Check sheet for the modelled part. Datum: model origin and axes. Units: mm. A direction names the side the tool comes from. Round coordinates to 2 decimals unless told otherwise and drop trailing zeros. Write each loop counter-clockwise with the first axis right and the second up, starting at its lowest first coordinate (ties: lowest second). Pieces come first, ordered by that corner, then holes.
Item 1: Material ranges on line 1 along Z through (x, y) = (-65, 16.75); line 2 along X through (y, z) = (6.5, -20.5); line 3 along X through (y, z) = (1, -19), recorded low to high.
Item 2: Set-up check for faces 4 (the flat face through (17, 7, -5)), 5 (the cylindrical face through (-70.198, 14.698, 16.524)), 6 (the flat face through (75, 15, -25)), 7 (the flat face through (-52, 15, 21.5)), 8 (the flat face through (-66, 16, 6)): record each of +Z, -Z, +X, -X, +Y, -Y from which the full face is reachable in a straight line by a thin tool's end or side.
Item 3: Section check C-C, the plane x = -20. Record the cut outline in (y, z), plus the area to 3 significant figures.
Item 4: Section check B-B, the plane y = 5.25. Record the cut outline in (x, z).
Item 5: Release check for a two-part mould opening along Z. For faces 1 (the flat face through (-66.5, 14, -13)), 2 (the cylindrical face through (99.948, 7.395, 16.128)), 3 (the flat face through (-18, 9, 26.5)) record: pulls with the +Z half, pulls with the -Z half, needs draft (parallel to the pull), parting line crosses it, or undercut.
Item 6: Section check A-A, the plane x = 1. Record the cut outline in (y, z).
Item 7: Depth check by flat-ended pin: pin 1 (9.5 mm diameter, centred on y = 17.5, z = 14.5, fed in from +X); pin 2 (5 mm diameter, centred on y = 13, z = 5.5, fed in from +X); pin 3 (10 mm diameter, centred on x = -6, y = 12.5, fed in from -Z). Enter the tip coordinate at first touch or a pass-through.
from build123d import *

# Parameters (mm, degrees)
BOSS_EXTRUDE1_DEPTH      = 10
SKETCH3_W                = 10
SKETCH3_H                = 17
BOSS_EXTRUDE2_DEPTH      = 12.5
RIB1_REACH               = 118.391
SKETCH4_WALL_W           = 271.329674284
SKETCH4_WALL_H           = 5
CUT_EXTRUDE1_REACH       = 170.771
SKETCH6_R                = 2.55
CUT_EXTRUDE2_DEPTH       = 2.5
BOSS_EXTRUDE4_DEPTH      = 5
BOSS_EXTRUDE4_DEPTH_BACK = 10
SKETCH11_R               = 30
CUT_EXTRUDE3_REACH       = 111.582
SKETCH8_R                = 14
CUT_EXTRUDE4_DEPTH       = 6
CUT_EXTRUDE4_DEPTH_BACK  = 7
SKETCH9_R                = 18.5
SKETCH12_R               = 24.5
CUT_EXTRUDE6_DEPTH       = 6
SKETCH13_R               = 2.05
CUT_EXTRUDE7_DEPTH       = 110.581884276
CUT_EXTRUDE9_START       = -2
SKETCH15_R               = 24.5
CUT_EXTRUDE9_DEPTH       = 2
SKETCH17_R               = 11.1
CUT_EXTRUDE11_DEPTH      = 7
CUT_EXTRUDE12_REACH      = 111.964
SKETCH18_R               = 4.5
SKETCH19_R               = 11.1
CUT_EXTRUDE13_DEPTH      = 7
CUT_EXTRUDE14_REACH      = 111.964
SKETCH20_R               = 4.5
SKETCH21_W               = 7
SKETCH21_H               = 3
BOSS_EXTRUDE5_DEPTH      = 7
SKETCH22_W               = 7
SKETCH22_H               = 2
BOSS_EXTRUDE6_DEPTH      = 5
SKETCH23_W               = 9.67527482
SKETCH23_H               = 3
BOSS_EXTRUDE7_DEPTH      = 8
SKETCH24_W               = 9.67527482
SKETCH24_H               = 2
BOSS_EXTRUDE8_DEPTH      = 3


with BuildPart() as part:
    # Sketch2 → Boss-Extrude1 (new body)
    with BuildSketch(Plane(origin=(0, 0, 0), x_dir=(1, 0, 0), z_dir=(0, 1, 0))):
        with BuildLine():
            Line((-74, 26.5), (74.6515139, 26.5))
            ThreePointArc((74.6515139, 26.5), (101.1515139, 0), (74.6515139, -26.5))
            Line((74.6515139, -26.5), (-74, -26.5))
            Line((-74, -26.5), (-74, 26.5))
        make_face()
    extrude(amount=BOSS_EXTRUDE1_DEPTH)

    # Sketch3 → Boss-Extrude2 (add)
    with BuildSketch(Plane(origin=(0, 10, 0), x_dir=(1, 0, 0), z_dir=(0, 1, 0))):
        with Locations((-69, -18)):
            Rectangle(SKETCH3_W, SKETCH3_H)
        with Locations((-69, 18)):
            Rectangle(SKETCH3_W, SKETCH3_H)
    extrude(amount=BOSS_EXTRUDE2_DEPTH)

    # Sketch4 wall → Rib1 (add, up to next)
    with BuildSketch(Plane(origin=(-46.828266128, 16.25, 26.5), x_dir=(0.939692620785, -0.342020143327, 0), z_dir=(0.342020143327, 0.939692620785, 0)), mode=Mode.PRIVATE) as rib1_sk1:
        with Locations((0, 2.5)):
            Rectangle(SKETCH4_WALL_W, SKETCH4_WALL_H)
    rib1_tool1 = extrude(rib1_sk1.sketch, amount=-RIB1_REACH, mode=Mode.PRIVATE) - part.part
    rib1 = rib1_tool1.solids().sort_by_distance((-46.828266128, 16.25, 26.5))[0]
    add(rib1)

    # Mirror1: Rib1 across plane
    add(rib1.mirror(Plane.XY))

    # Sketch6 → Cut-Extrude1 (cut, up to next)
    with BuildSketch(Plane(origin=(-64, 0, 0), x_dir=(0, 0, -1), z_dir=(1, 0, 0)), mode=Mode.PRIVATE) as cut_extrude1_sk1:
        with Locations((-14.5, 16.25)):
            Circle(SKETCH6_R)
    cut_extrude1_tool1 = extrude(cut_extrude1_sk1.sketch, amount=-CUT_EXTRUDE1_REACH, mode=Mode.PRIVATE) & part.part
    cut_extrude1 = cut_extrude1_tool1.solids().sort_by_distance((-64, 16.25, 14.5))[0]
    add(cut_extrude1, mode=Mode.SUBTRACT)

    # Sketch7 → Cut-Extrude2 (cut)
    with BuildSketch(Plane(origin=(-64, 0, 0), x_dir=(0, 0, -1), z_dir=(1, 0, 0))):
        Polygon((-10.45, 13.91173141), (-10.45, 18.58826859), (-14.5, 20.92653718), (-18.55, 18.58826859), (-18.55, 13.91173141), (-14.5, 11.57346282), align=None)
    cut_extrude2 = extrude(amount=-CUT_EXTRUDE2_DEPTH, mode=Mode.SUBTRACT)

    # Mirror2: Cut-Extrude1, Cut-Extrude2 across plane
    add(cut_extrude1.mirror(Plane.XY), mode=Mode.SUBTRACT)
    add(cut_extrude2.mirror(Plane.XY), mode=Mode.SUBTRACT)

    # Sketch11 → Boss-Extrude4 (add, two sides: drawn at the far end of the back side and taken through both)
    with BuildSketch(Plane(origin=(0, 10, 0), x_dir=(1, 0, 0), z_dir=(0, 1, 0)).offset(-BOSS_EXTRUDE4_DEPTH_BACK)):
        with Locations(Location((74.6515139, 0, 0), (0, 0, 270))):
            Circle(SKETCH11_R)
    extrude(amount=BOSS_EXTRUDE4_DEPTH + BOSS_EXTRUDE4_DEPTH_BACK)

    # Sketch8 → Cut-Extrude3 (cut, up to next)
    with BuildSketch(Plane(origin=(0, 10, 0), x_dir=(1, 0, 0), z_dir=(0, 1, 0)), mode=Mode.PRIVATE) as cut_extrude3_sk1:
        with Locations(Location((74.6515139, 0, 0), (0, 0, 270))):
            Circle(SKETCH8_R)
    cut_extrude3_tool1 = extrude(cut_extrude3_sk1.sketch, amount=-CUT_EXTRUDE3_REACH, mode=Mode.PRIVATE) & part.part
    add(cut_extrude3_tool1.solids().sort_by_distance((74.651514, 10, 0))[0], mode=Mode.SUBTRACT)

    # Sketch9 → Cut-Extrude4 (cut, two sides: drawn at the far end of the back side and taken through both)
    with BuildSketch(Plane(origin=(0, 10, 0), x_dir=(1, 0, 0), z_dir=(0, 1, 0)).offset(-CUT_EXTRUDE4_DEPTH_BACK)):
        with Locations(Location((74.6515139, 0, 0), (0, 0, 270))):
            Circle(SKETCH9_R)
    extrude(amount=CUT_EXTRUDE4_DEPTH + CUT_EXTRUDE4_DEPTH_BACK, mode=Mode.SUBTRACT)

    # Sketch12 → Cut-Extrude6 (cut)
    with BuildSketch(Plane(origin=(0, 15, 0), x_dir=(1, 0, 0), z_dir=(0, 1, 0))):
        with Locations(Location((74.6515139, 0, 0), (0, 0, 270))):
            Circle(SKETCH12_R)
    extrude(amount=-CUT_EXTRUDE6_DEPTH, mode=Mode.SUBTRACT)

    # Sketch13 → Cut-Extrude7 (cut, through all)
    with BuildSketch(Plane(origin=(0, 10, 0), x_dir=(1, 0, 0), z_dir=(0, 1, 0))):
        with Locations(Location((1, -20.5, 0), (0, 0, 270))):
            Circle(SKETCH13_R)
        with Locations(Location((31, -20.5, 0), (0, 0, 270))):
            Circle(SKETCH13_R)
    cut_extrude7 = extrude(amount=-CUT_EXTRUDE7_DEPTH, mode=Mode.SUBTRACT)

    # Sketch15 → Cut-Extrude9 (cut)
    with BuildSketch(Plane.XZ.offset(CUT_EXTRUDE9_START)):
        with Locations(Location((74.6515139, 0, 0), (0, 0, 90))):
            Circle(SKETCH15_R)
    extrude(amount=CUT_EXTRUDE9_DEPTH, mode=Mode.SUBTRACT)

    # Sketch17 → Cut-Extrude11 (cut)
    with BuildSketch(Plane.XZ):
        with Locations(Location((-40.5, 0, 0), (0, 0, 270))):
            Circle(SKETCH17_R)
    extrude(amount=-CUT_EXTRUDE11_DEPTH, mode=Mode.SUBTRACT)

    # Sketch18 → Cut-Extrude12 (cut, up to next)
    with BuildSketch(Plane.XZ.offset(-7), mode=Mode.PRIVATE) as cut_extrude12_sk1:
        with Locations(Location((-40.5, 0, 0), (0, 0, 270))):
            Circle(SKETCH18_R)
    cut_extrude12_tool1 = extrude(cut_extrude12_sk1.sketch, amount=-CUT_EXTRUDE12_REACH, mode=Mode.PRIVATE) & part.part
    add(cut_extrude12_tool1.solids().sort_by_distance((-40.5, 7, 0))[0], mode=Mode.SUBTRACT)

    # Sketch19 → Cut-Extrude13 (cut)
    with BuildSketch(Plane.XZ):
        with Locations(Location((17, 0, 0), (0, 0, 270))):
            Circle(SKETCH19_R)
    extrude(amount=-CUT_EXTRUDE13_DEPTH, mode=Mode.SUBTRACT)

    # Sketch20 → Cut-Extrude14 (cut, up to next)
    with BuildSketch(Plane.XZ.offset(-7), mode=Mode.PRIVATE) as cut_extrude14_sk1:
        with Locations(Location((17, 0, 0), (0, 0, 270))):
            Circle(SKETCH20_R)
    cut_extrude14_tool1 = extrude(cut_extrude14_sk1.sketch, amount=-CUT_EXTRUDE14_REACH, mode=Mode.PRIVATE) & part.part
    add(cut_extrude14_tool1.solids().sort_by_distance((17, 7, 0))[0], mode=Mode.SUBTRACT)

    # Mirror3: Cut-Extrude7 across plane
    add(cut_extrude7.mirror(Plane.XY), mode=Mode.SUBTRACT)

    # Sketch21 → Boss-Extrude5 (add)
    with BuildSketch(Plane(origin=(0, 10, 0), x_dir=(1, 0, 0), z_dir=(0, 1, 0))):
        with Locations((-45.5, -13)):
            Rectangle(SKETCH21_W, SKETCH21_H)
    extrude(amount=BOSS_EXTRUDE5_DEPTH)

    # Sketch22 → Boss-Extrude6 (add)
    with BuildSketch(Plane.XY.offset(14.5)):
        with Locations((-45.5, 16)):
            Rectangle(SKETCH22_W, SKETCH22_H)
    extrude(amount=BOSS_EXTRUDE6_DEPTH)

    # Sketch23 → Boss-Extrude7 (add)
    with BuildSketch(Plane(origin=(0, 10, 0), x_dir=(1, 0, 0), z_dir=(0, 1, 0))):
        with Locations((-65.857730682, -3)):
            Rectangle(SKETCH23_W, SKETCH23_H)
    extrude(amount=BOSS_EXTRUDE7_DEPTH)

    # Sketch24 → Boss-Extrude8 (add)
    with BuildSketch(Plane.XY.offset(4.5)):
        with Locations((-65.857730682, 17)):
            Rectangle(SKETCH24_W, SKETCH24_H)
    extrude(amount=BOSS_EXTRUDE8_DEPTH)


solid = part.part
Values found:
1. line 1: z = -26.5 to -18.55, -10.45 to -9.5, 1.5 to 7.5, 9.5 to 10.45, 18.55 to 26.5
1. line 2: x = -74 to -1.05, 3.05 to 28.95, 33.05 to 96.55
1. line 3: x = -74 to -0.4, 2.4 to 29.6, 32.4 to 59.18, 90.12 to 97.87
2. face 4: -Y
2. face 5: -X
2. face 6: +Z, -Z, +X, +Y
2. face 7: +Y
2. face 8: +X, -X
3. outline: (0, -26.5) - (10, -26.5) - (10, 26.5) - (0, 26.5) - close
3. area: 530 mm2
4. outline: (-74, -26.5) - (60.59, -26.5) arc R30 ccw (long way) to (60.59, 26.5) - (-74, 26.5) - close; hole circle Ø22.2 at (-40.5, 0); hole circle Ø4.1 at (1, -20.5); hole circle Ø4.1 at (1, 20.5); hole circle Ø22.2 at (17, 0); hole circle Ø4.1 at (31, -20.5); hole circle Ø4.1 at (31, 20.5); hole circle Ø37 at (74.65, 0)
5. face 1: undercut
5. face 2: parting line crosses it
5. face 3: pulls with the +Z half
6. outline: (0, -26.5) - (10, -26.5) - (10, -22.55) - (0, -22.55) - close; (0, -18.45) - (10, -18.45) - (10, 18.45) - (0, 18.45) - close; (0, 22.55) - (10, 22.55) - (10, 26.5) - (0, 26.5) - close
7. pin 1: stops at x = 102.77
7. pin 2: stops at x = 104.5
7. pin 3: stops at z = -26.5
